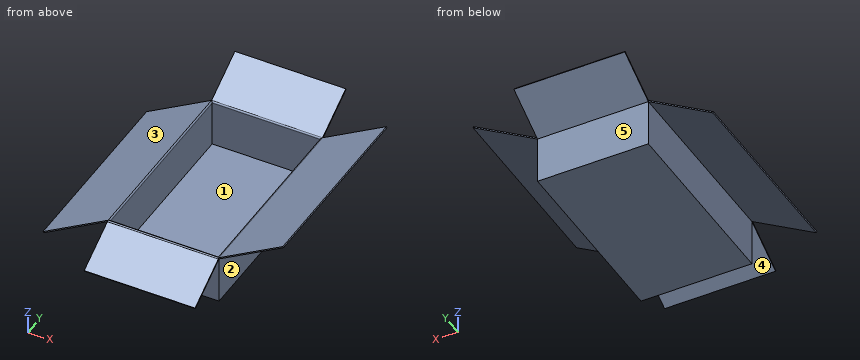
```python
from build123d import *

# Parameters (mm, degrees)
F0_W     = 268
F0_H     = 115
F1_DEPTH = 463.5
F2_T     = -3
F4_DEPTH = 463.5
F6_DEPTH = 268


with BuildPart() as f1:
    # F0 (on Front) → F1 (new body)
    with BuildSketch(Plane.XZ):
        with Locations((134, 57.5)):
            Rectangle(F0_W, F0_H)
    extrude(amount=F1_DEPTH)

    # F2
    f2_openings = [f1.faces().sort_by_distance(p)[0] for p in [
        (134, -231.75, 115),
    ]]
    offset(amount=F2_T, openings=f2_openings)

    # F3 (on face) → F4 (join, through all)
    with BuildSketch(Plane.XZ.offset(463.5)):
        with BuildLine():
            Line((-155.884573, 25), (0, 115))
            Line((0, 115), (3.464102, 115))
            ThreePointArc((3.464102, 115), (2.44949, 117.44949), (0, 118.464102))
            Line((0, 118.464102), (-157.384573, 27.598076))
            Line((-157.384573, 27.598076), (-155.884573, 25))
        make_face()
        with BuildLine():
            Line((264.535898, 115), (268, 115))
            Line((268, 115), (423.884573, 205))
            Line((423.884573, 205), (422.384573, 207.598076))
            Line((422.384573, 207.598076), (268, 118.464102))
            ThreePointArc((268, 118.464102), (265.55051, 117.44949), (264.535898, 115))
        make_face()
    extrude(amount=-F4_DEPTH)

    # F5 (on face) → F6 (join, through all)
    with BuildSketch(Plane(origin=(0, 0, 0), x_dir=(0, -1, 0), z_dir=(-1, 0, 0))):
        with BuildLine():
            Line((460.035898, 115), (463.5, 115))
            Line((463.5, 115), (569.155099, 54))
            Line((569.155099, 54), (570.655099, 56.598076))
            Line((570.655099, 56.598076), (466.5, 116.732051))
            ThreePointArc((466.5, 116.732051), (465.232051, 118), (463.5, 118.464102))
            ThreePointArc((463.5, 118.464102), (461.05051, 117.44949), (460.035898, 115))
        make_face()
        with BuildLine():
            Line((-105.655099, 176), (0, 115))
            Line((0, 115), (3.464102, 115))
            ThreePointArc((3.464102, 115), (2.44949, 117.44949), (0, 118.464102))
            Line((0, 118.464102), (-104.155099, 178.598076))
            Line((-104.155099, 178.598076), (-105.655099, 176))
        make_face()
    extrude(amount=-F6_DEPTH)


solid = f1.part
```
Could you check a few things on this model? Use its own coordinates, in mm. Face numbers are marked on the shaded views. A direction names the side the tool comes from. Give positions to 0.01 mm unless a question says otherwise; leave off trailing zeros. Order: outer loops, then holes, each group sorted by start corner. A loop starts at its lowest first (then second) coordinate and runs counter-clockwise, first axis right, second up.
Q1. For the marked faces 4 and 5, which set-ups out of +Z, -Z, +X, -X, +Y, -Y let a thin tool reach every point of the face, with its end or its side?
Q2. We'd pull the mould along X, two halves only. Please class the marked faces 1, 2 and 3: +X half, -X half, draft (parallel to the pull), parting line (faces both ways), or undercut.
Q3. I'm going to push flat-ended pins straight in: P1, Ø19.5, axis at y = -536, z = 72, coming from the -X side; P2, Ø4, axis at y = -298, z = 55, coming from the -X side; P3, Ø5, axis at y = -415.5, z = 64, coming from the +X side. Where does each tip first touch, or does it pass through?
Q4. Suppose I cut it at A-A, the plane x = 118. Write out the boundary of the cut face in (y, z).
Q5. Suppose I cut it at B-B, the plane z = 96. Write out the boundary of the cut face in (x, y).
Q6. If I drill on line 1 along X through (y, z) = (-59, 33.5); line 2 along Y through (x, z) = (74, 18.5); line 3 along X through (y, z) = (-177.5, 59), over which ranges is the centre line in solid material (lowest first)?
Q7. Suppose I cut it at D-D, the plane z = 17. Write out the boundary of the cut face in (x, y), and give its area (3 significant figures).
Q8. Suppose I cut it at C-C, the plane y = -180. Write out the boundary of the cut face in (x, z), and give its area (3 significant figures).
Solution:
1. face 4: -Z, +X, -X
1. face 5: -Z, +X, -X, +Y
2. face 1: undercut
2. face 2: +X half
2. face 3: -X half
3. P1: stops at x = 0
3. P2: stops at x = -113.39
3. P3: stops at x = 268
4. outline: (-570.66, 56.6) - (-569.16, 54) - (-463.5, 115) - (-463.5, 0) - (0, 0) - (0, 115) - (105.66, 176) - (104.16, 178.6) - (0, 118.46) arc R3.46 ccw to (-3.46, 115) - (-3, 115) - (-3, 3) - (-460.5, 3) - (-460.5, 115) - (-460.04, 115) arc R3.46 ccw to (-466.5, 116.73) - close
5. outline: (-38.91, -463.5) - (-32.91, -463.5) - (-32.91, 0) - (-38.91, 0) - close; (0, -502.41) - (268, -502.41) - (268, -496.41) - (0, -496.41) - close; (0, -463.5) - (268, -463.5) - (268, 0) - (0, 0) - close; hole (3, -460.5) - (265, -460.5) - (265, -3) - (3, -3) - close
6. line 1: x = -147.16 to -141.16, 0 to 3, 265 to 268
6. line 2: y = -463.5 to -460.5, -3 to 0
6. line 3: x = -102.99 to -96.99, 0 to 3, 265 to 268
7. outline: (0, -463.5) - (268, -463.5) - (268, 0) - (0, 0) - close; hole (3, -460.5) - (265, -460.5) - (265, -3) - (3, -3) - close
7. area: 4,350 mm2
8. outline: (-157.38, 27.6) - (-155.88, 25) - (0, 115) - (0, 0) - (268, 0) - (268, 115) - (423.88, 205) - (422.38, 207.6) - (268, 118.46) arc R3.46 ccw to (264.54, 115) - (265, 115) - (265, 3) - (3, 3) - (3, 115) - (3.46, 115) arc R3.46 ccw to (0, 118.46) - close
8. area: 2,570 mm2
